from build123d import *

# Parameters (mm, degrees)
SKETCH_1_R      = 8
SKETCH_1_R_2    = 2.5
EXTRUDE_1_DEPTH = 1
SKETCH_2_R      = 6
SKETCH_2_R_2    = 2.5
EXTRUDE_2_DEPTH = 6.5
SKETCH_3_R      = 8
SKETCH_3_R_2    = 6
EXTRUDE_3_DEPTH = 1
SKETCH_4_R      = 6
SKETCH_4_R_2    = 2.5
EXTRUDE_4_DEPTH = 1


with BuildPart() as part:
    # Sketch 1 → Extrude 1 (new body)
    with BuildSketch(Plane.XY):
        Circle(SKETCH_1_R)
        Circle(SKETCH_1_R_2, mode=Mode.SUBTRACT)
    extrude(amount=EXTRUDE_1_DEPTH)

    # Sketch 2 → Extrude 2 (add)
    with BuildSketch(Plane.XY.offset(1)):
        with Locations(Location((0, 0, 0), (0, 0, 180))):
            Circle(SKETCH_2_R)
        Circle(SKETCH_2_R_2, mode=Mode.SUBTRACT)
    extrude(amount=EXTRUDE_2_DEPTH)



with BuildPart() as body_2:
    # Sketch 3 → Extrude 3 (new body)
    with BuildSketch(Plane.XY.offset(7.5)):
        Circle(SKETCH_3_R)
        with Locations(Location((0, 0, 0), (0, 0, 180))):
            Circle(SKETCH_3_R_2, mode=Mode.SUBTRACT)
    extrude(amount=EXTRUDE_3_DEPTH)


with BuildPart() as part_1:
    add(part.part)

    add(body_2.part)  # Extrude 4 merges body 2
    # Sketch 4 → Extrude 4 (add)
    with BuildSketch(Plane.XY.offset(7.5)):
        with Locations(Location((0, 0, 0), (0, 0, 180))):
            Circle(SKETCH_4_R)
        Circle(SKETCH_4_R_2, mode=Mode.SUBTRACT)
    extrude(amount=EXTRUDE_4_DEPTH)


solid = part_1.part
The listing builds one solid part. Answer for the finished solid, in the listing's coordinates (mm). A direction names the side the tool comes from. Coordinates: 2 decimals unless noted, no trailing zeros. Write each loop counter-clockwise with the first axis right and the second up, starting at its lowest first coordinate (ties: lowest second). Pieces come first, ordered by that corner, then holes. Notation, with made-up numbers: (66.25, -14) - (72.25, -14) arc R15 cw to (72.25, -6) - close; hole circle Ø10 at (-13.75, -7). An arc over 180 degrees is marked (long way). Return JSON: item names as keys, results as strings.
1. Which of the six approach directions +Z, -Z, +X, -X, +Y, -Y give full straight-line access (tool end or side, diameter ignored) to faces 4 (the face through (-0.54, -2.44, 4.19)), 5 (the face through (-5.723, -1.802, 4.204))?
Final values:
{"face 4": "+Z, -Z", "face 5": "none"}
2. For a pull along Z with two mould halves and no side action, classify faces 1 (the face through (-1.73, -7.81, 7.99)), 2 (the face through (-2, -2, 8.5)), 3 (the face through (-2, 6, 7.5)) as +Z half, -Z half, draft (parallel to the pull), parting line (faces both ways), or undercut.
Final values:
{"face 1": "draft", "face 2": "+Z half", "face 3": "undercut"}
3. The part is cut by section D-D on x = 5.5. Determine the outline of the cut face in (y, z), then the cut area to 3 significant figures.
Final values:
{"outline": "(-5.81, 0) - (5.81, 0) - (5.81, 1) - (2.4, 1) - (2.4, 7.5) - (5.81, 7.5) - (5.81, 8.5) - (-5.81, 8.5) - (-5.81, 7.5) - (-2.4, 7.5) - (-2.4, 1) - (-5.81, 1) - close", "area": "54.4 mm^2"}
4. The part is cut by section A-A on y = 0. Determine the outline of the cut face in (x, z), then the cut area to 3 significant figures.
Final values:
{"outline": "(-8, 0) - (-2.5, 0) - (-2.5, 8.5) - (-8, 8.5) - (-8, 7.5) - (-6, 7.5) - (-6, 1) - (-8, 1) - close; (2.5, 0) - (8, 0) - (8, 1) - (6, 1) - (6, 7.5) - (8, 7.5) - (8, 8.5) - (2.5, 8.5) - close", "area": "67.5 mm^2"}
5. Consider line 1 along Z through (x, y) = (6, -5.25); line 2 along Y through (x, z) = (0, 4.25); line 3 along X through (y, z) = (-0.5, 3.75). Determine where each line is inside the solid, lowest interval first.
Final values:
{"line 1": "0 to 1, 7.5 to 8.5", "line 2": "-6 to -2.5, 2.5 to 6", "line 3": "-5.98 to -2.45, 2.45 to 5.98"}
6. The part is cut by section C-C on z = 1.25. Determine the outline of the cut face in (x, y).
Final values:
{"outline": "circle Ø12 at (0, 0); hole circle Ø5 at (0, 0)"}
7. Each of these flat-tipped pins is pushed along its axis until it touches: pin 1 Ø3 at (y, z) = (4, 6.5) entering from -X; pin 2 Ø4 at (y, z) = (6.5, 4.5) entering from -X; pin 3 Ø1 at (x, z) = (-4, 4) entering from +Y. Where does it stop, or does it pass through?
Final values:
{"pin 1": "x = -7.46", "pin 2": "x = -3.97", "pin 3": "y = 4.87"}
